Part model, mm, in its own coordinate system. Face numbers are marked on the shaded views. A direction names the side the tool comes from. Round coordinates to 2 decimals unless told otherwise and drop trailing zeros. Loops run counter-clockwise (first coordinate to the right, second up) from the corner with the lowest first, then second, coordinate; pieces in that order, holes last. Notation, with made-up numbers: M -39.75,17.25 L -18.75,17.25 A20 cw -18.75,36.25 Z; hole C -14,64.5 d8. An arc over 180 degrees is marked long. Answer as CSV lines item,"result". Start each with the question number.
Item 1: Band-saw the part on C-C (x = -70). Give the cut face in (y, z).
Item 2: Wall check: line 1 (Y direction, x = -73.85, z = 13.75); line 2 (Z direction, x = -56.5, y = -70); line 3 (Y direction, x = -62.75, z = 28.25). Give the ranges that are in metal, low to high.
Item 3: Drop a flat-ended pin along its axis: pin 1 Ø6 at (y, z) = (-34.5, 13.5) entering from +X. Give the stop position or say it passes through.
Item 4: Band-saw the part on B-B (z = 12.25). Give the cut face in (x, y), and give its area (3 significant figures).
Item 5: Mould opens along Z. For the marked faces 3, 4, 5 and 6 say: pulls with the +Z half, pulls with the -Z half, needs draft (parallel to the pull), parting line crosses it, or undercut.
Item 6: Band-saw the part on A-A (y = -120). Give the cut face in (x, z).
Item 7: Band-saw the part on D-D (y = -80). Give the cut face in (x, z), and give its area (4 significant figures).
Item 8: Which spindle directions (+Z, -Z, +X, -X, +Y, -Y) get a long thin tool onto all of the face, cutting with end or side? Do the marked faces 1 and 2. Say none if no direction does.
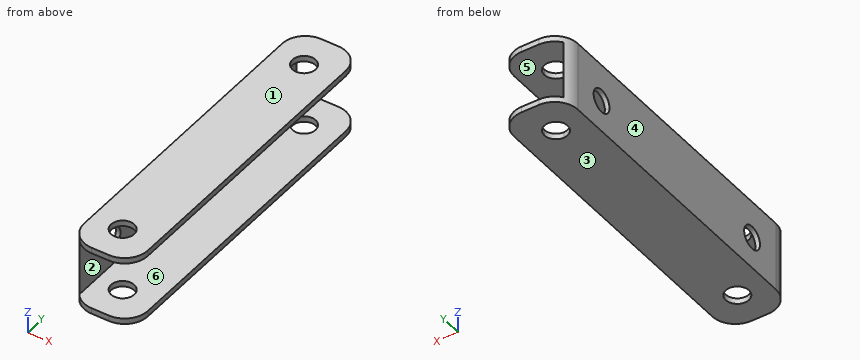
```python
from build123d import *

# Parameters (mm, degrees)
F2_DEPTH    = 145
F1_R        = 5
F3_DEPTH    = 46
F4_T1_DEPTH = 52.5
F4_T3_DEPTH = 52.5
F4_T5_DEPTH = 80
F7_DEPTH    = 25


# Not quite as in the source:
# - a fillet or chamfer that OpenCascade refuses, or shapes differently, is made with other operations: its cross-section is extruded or revolved along the edge and cut away or added


with BuildPart() as f2:
    # F0 (on Front) → F2 (new body)
    with BuildSketch(Plane.XZ):
        Polygon((-74.9858543277, 30), (-74.9858543277, 0), (-47.4858543277, 0), (-47.4858543277, 2.5), (-72.9858543277, 2.5), (-72.9858543277, 27.5), (-47.4858543277, 27.5), (-47.4858543277, 30), align=None)
    extrude(amount=F2_DEPTH)

    # F1 (on Top) → F3 (cut)
    with BuildSketch(Plane.XY):
        with BuildLine():
            ThreePointArc((-59.9858543277, -290), (-54.9858543277, -295), (-49.9858543277, -290))
            ThreePointArc((-49.9858543277, -290), (-54.9858543277, -285), (-59.9858543277, -290))
        make_face()
        with Locations((-54.9858543277, -260)):
            Circle(F1_R)
        with Locations((-61.7693625391, -129.9988627434)):
            Circle(F1_R)
        with BuildLine():
            ThreePointArc((-61.7693625391, -20.5436318724), (-58.2338286331, -19.0791657783), (-56.7693625391, -15.5436318724))
            ThreePointArc((-56.7693625391, -15.5436318724), (-65.304896445, -12.0080979665), (-61.7693625391, -20.5436318724))
        make_face()
    extrude(amount=F3_DEPTH, mode=Mode.SUBTRACT)

    # F4: fillet of radius 10 on 6 edges, made by hand

    # F4_s2 → F4_t1 (cut)
    with BuildSketch(Plane.XY.offset(-25)):
        with BuildLine():
            ThreePointArc((-57.4858543277, 0), (-50.4147865158, -2.9289321881), (-47.4858543277, -10))
            Line((-47.4858543277, -10), (-47.4858543277, 0))
            Line((-47.4858543277, 0), (-57.4858543277, 0))
        make_face()
        with BuildLine():
            ThreePointArc((-57.4858543277, -145), (-50.4147865158, -142.0710678119), (-47.4858543277, -135))
            Line((-47.4858543277, -135), (-47.4858543277, -145))
            Line((-47.4858543277, -145), (-57.4858543277, -145))
        make_face()
    extrude(amount=F4_T1_DEPTH, mode=Mode.SUBTRACT)

    # F4_s4 → F4_t3 (cut)
    with BuildSketch(Plane.XY.offset(2.5)):
        with BuildLine():
            ThreePointArc((-47.4858543277, -10), (-50.4147865158, -2.9289321881), (-57.4858543277, 0))
            Line((-57.4858543277, 0), (-47.4858543277, 0))
            Line((-47.4858543277, 0), (-47.4858543277, -10))
        make_face()
        with BuildLine():
            ThreePointArc((-47.4858543277, -135), (-50.4147865158, -142.0710678119), (-57.4858543277, -145))
            Line((-57.4858543277, -145), (-47.4858543277, -145))
            Line((-47.4858543277, -145), (-47.4858543277, -135))
        make_face()
    extrude(amount=F4_T3_DEPTH, mode=Mode.SUBTRACT)

    # F4_s6 → F4_t5 (cut)
    with BuildSketch(Plane.XY.offset(-25)):
        with BuildLine():
            ThreePointArc((-64.9858543277, 0), (-72.0569221395, -2.9289321881), (-74.9858543277, -10))
            Line((-74.9858543277, -10), (-74.9858543277, 0))
            Line((-74.9858543277, 0), (-64.9858543277, 0))
        make_face()
        with BuildLine():
            ThreePointArc((-64.9858543277, -145), (-72.0569221395, -142.0710678119), (-74.9858543277, -135))
            Line((-74.9858543277, -135), (-74.9858543277, -145))
            Line((-74.9858543277, -145), (-64.9858543277, -145))
        make_face()
    extrude(amount=F4_T5_DEPTH, mode=Mode.SUBTRACT)

    # F6 (on offset) → F7 (cut)
    with BuildSketch(Plane(origin=(-74.9858543277, 0, 0), x_dir=(0, -1, 0), z_dir=(-1, 0, 0))):
        with BuildLine():
            ThreePointArc((30, 13.75), (21.4644660941, 17.2855339059), (25, 8.75))
            Line((25, 8.75), (25, 13.75))
            Line((25, 13.75), (30, 13.75))
        make_face()
        with BuildLine():
            Line((25, 13.75), (25, 8.75))
            ThreePointArc((25, 8.75), (28.5355339059, 10.2144660941), (30, 13.75))
            Line((30, 13.75), (25, 13.75))
        make_face()
        with BuildLine():
            Line((120, 13.75), (125, 13.75))
            ThreePointArc((125, 13.75), (120, 18.75), (115, 13.75))
            Line((115, 13.75), (120, 13.75))
        make_face()
        with BuildLine():
            ThreePointArc((115, 13.75), (120, 8.75), (125, 13.75))
            Line((125, 13.75), (120, 13.75))
            Line((120, 13.75), (115, 13.75))
        make_face()
    extrude(amount=-F7_DEPTH, mode=Mode.SUBTRACT)


solid = f2.part
```
Answer block:
1,outline,"M -143.65,0 L -1.35,0 L -1.35,2.5 L -143.65,2.5 Z; M -143.65,27.5 L -1.35,27.5 L -1.35,30 L -143.65,30 Z"
2,line 1,"y = -139.63 to -125, -115 to -30, -20 to -5.37"
2,line 2,"z = 0 to 2.5, 27.5 to 30"
2,line 3,"y = -145 to -134.9, -125.1 to -20.45, -10.64 to 0"
3,pin 1,"stops at x = -72.99"
4,outline,"M -74.99,-135 A10 ccw -72.99,-141 L -72.99,-124.77 L -74.99,-124.77 Z; M -74.99,-115.23 L -72.99,-115.23 L -72.99,-29.77 L -74.99,-29.77 Z; M -74.99,-20.23 L -72.99,-20.23 L -72.99,-4 A10 ccw -74.99,-10 Z"
4,area,"228 mm^2"
5,face 3,"pulls with the -Z half"
5,face 4,"needs draft"
5,face 5,"undercut"
5,face 6,"undercut"
6,outline,"M -74.99,0 L -47.49,0 L -47.49,2.5 L -72.99,2.5 L -72.99,8.75 L -74.99,8.75 Z; M -74.99,18.75 L -72.99,18.75 L -72.99,27.5 L -47.49,27.5 L -47.49,30 L -74.99,30 Z"
7,outline,"M -74.99,0 L -47.49,0 L -47.49,2.5 L -72.99,2.5 L -72.99,27.5 L -47.49,27.5 L -47.49,30 L -74.99,30 Z"
7,area,"187.5 mm^2"
8,face 1,"+Z, +X, -X, +Y, -Y"
8,face 2,"+X, +Y, -Y"
